```python
from build123d import *

# Parameters (mm, degrees)
SKETCH_W            = 85
SKETCH_H            = 190
PAD_DEPTH           = 1
SKETCH001_W         = 2
SKETCH001_H         = 50
PAD001_DEPTH        = 190
SKETCH002_W         = 2
SKETCH002_H         = 50
PAD002_DEPTH        = 85
SKETCH003_W         = 2
SKETCH003_H         = 50
PAD003_DEPTH        = 85
SKETCH004_W         = 2
SKETCH004_H         = 5
PAD004_DEPTH        = 190
POCKET_DEPTH        = 2
POCKET001_DEPTH     = 190
POCKET002_DEPTH     = 2
LINEARPATTERN_COUNT = 3
LINEARPATTERN_PITCH = 85


with BuildPart() as part:
    # Sketch → Pad (new body)
    with BuildSketch(Plane.XY):
        with Locations((-42.5, 95)):
            Rectangle(SKETCH_W, SKETCH_H)
    extrude(amount=PAD_DEPTH)

    # Sketch001 → Pad001 (join)
    with BuildSketch(Plane.XZ):
        with Locations((-1, 25)):
            Rectangle(SKETCH001_W, SKETCH001_H)
    extrude(amount=-PAD001_DEPTH)

    # Sketch002 → Pad002 (join)
    with BuildSketch(Plane.YZ):
        with Locations((1, 25)):
            Rectangle(SKETCH002_W, SKETCH002_H)
    extrude(amount=-PAD002_DEPTH)

    # Sketch003 → Pad003 (join)
    with BuildSketch(Plane.YZ):
        with Locations((189, 25)):
            Rectangle(SKETCH003_W, SKETCH003_H)
    extrude(amount=-PAD003_DEPTH)

    # Sketch004 → Pad004 (join)
    with BuildSketch(Plane.XZ):
        with Locations((-84, 2.5)):
            Rectangle(SKETCH004_W, SKETCH004_H)
    extrude(amount=-PAD004_DEPTH)

    # Sketch005 → Pocket (cut)
    with BuildSketch(Plane.XZ):
        with BuildLine():
            ThreePointArc((-7, 6.5), (-8.5, 5), (-7, 3.5))
            Line((-7, 3.5), (-5, 3.5))
            ThreePointArc((-5, 3.5), (-3.5, 5), (-5, 6.5))
            Line((-7, 6.5), (-5, 6.5))
        make_face()
    extrude(amount=-POCKET_DEPTH, mode=Mode.SUBTRACT)

    # Sketch006 → Pocket001 (cut)
    with BuildSketch(Plane.XZ):
        with BuildLine():
            ThreePointArc((-12, 46.6), (-13.6, 45), (-12, 43.4))
            Line((-12, 43.4), (-10, 43.4))
            ThreePointArc((-10, 43.4), (-8.4, 45), (-10, 46.6))
            Line((-12, 46.6), (-10, 46.6))
        make_face()
        with BuildLine():
            ThreePointArc((-77, 46.6), (-78.6, 45), (-77, 43.4))
            Line((-77, 43.4), (-75, 43.4))
            ThreePointArc((-75, 43.4), (-73.4, 45), (-75, 46.6))
            Line((-77, 46.6), (-75, 46.6))
        make_face()
    extrude(amount=-POCKET001_DEPTH, mode=Mode.SUBTRACT)

    # Sketch007 → Pocket002 (cut)
    with BuildSketch(Plane.YZ):
        with BuildLine():
            ThreePointArc((10, 46.6), (8.4, 45), (10, 43.4))
            Line((10, 43.4), (12, 43.4))
            ThreePointArc((12, 43.4), (13.6, 45), (12, 46.6))
            Line((10, 46.6), (12, 46.6))
        make_face()
    pocket002 = extrude(amount=-POCKET002_DEPTH, mode=Mode.SUBTRACT)

    # LinearPattern: Pocket002 ×3
    with Locations(*[(0, i * LINEARPATTERN_PITCH, 0) for i in range(1, LINEARPATTERN_COUNT)]):
        add(pocket002, mode=Mode.SUBTRACT)


solid = part.part
```
Geometry check sheet. Reference: the model listing, model coordinates, mm. Give positions to 0.01 mm unless a question says otherwise; leave off trailing zeros. Write each loop counter-clockwise with the first axis right and the second up, starting at its lowest first coordinate (ties: lowest second). Pieces come first, ordered by that corner, then holes.
1) Section check A-A, the plane y = 113. Record the boundary of the cut face in (x, z), and give its area (3 significant figures).
2) Section check B-B, the plane z = 29. Record the boundary of the cut face in (x, y).
3) Gauge pin test, flat ends, axial feed: pin 1 (10 mm diameter, centred on x = -60.5, y = 168.5, fed in from -Z); pin 2 (1.6 mm diameter, centred on x = -84, y = 129, fed in from +Z); pin 3 (12 mm diameter, centred on x = -55.5, y = 133, fed in from +Z); pin 4 (1.5 mm diameter, centred on y = 57, z = 44, fed in from -X). Record the tip position at first contact, or that the pin passes through.
4) Material ranges on L1, parallel to Y at x = -4, z = 25; L2, parallel to X at y = 132, z = 3; L3, parallel to Z at x = -68.5, y = 157, recorded low to high.
5) Release check for a two-part mould opening along X. For faces 1 (the flat face through (0, 94, 25)), 2 (the flat face through (-43, 96, 1)), 3 (the flat face through (-83, 94, 3)), 4 (the flat face through (-43, 0, 25)) record: pulls with the +X half, pulls with the -X half, needs draft (parallel to the pull), parting line crosses it, or undercut.
Computed:
1. outline: (-85, 0) - (0, 0) - (0, 50) - (-2, 50) - (-2, 1) - (-83, 1) - (-83, 5) - (-85, 5) - close
1. area: 191 mm2
2. outline: (-85, 0) - (0, 0) - (0, 190) - (-85, 190) - (-85, 188) - (-2, 188) - (-2, 2) - (-85, 2) - close
3. pin 1: stops at z = 0
3. pin 2: stops at z = 5
3. pin 3: stops at z = 1
3. pin 4: stops at x = -2
4. L1: y = 0 to 2, 188 to 190
4. L2: x = -85 to -83, -2 to 0
4. L3: z = 0 to 1
5. face 1: pulls with the +X half
5. face 2: undercut
5. face 3: undercut
5. face 4: needs draft
